CAD build for the part. Positions are in the model's coordinates, mm. A direction names the side the tool comes from. Round coordinates to 2 decimals unless told otherwise and drop trailing zeros. Loops run counter-clockwise (first coordinate to the right, second up) from the corner with the lowest first, then second, coordinate; pieces in that order, holes last.
```python
from build123d import *

# Parameters (mm, degrees)
F0_W      = 73.406
F0_H      = 31.75
F1_DEPTH  = 14.224
F3_DEPTH  = 28.575
F5_DEPTH  = 25.4
F8_DEPTH  = 12.7
F10_DEPTH = 4.826
F12_DEPTH = 4.826


with BuildPart() as f1:
    # F0 (on Front) → F1 (new body, symmetric)
    with BuildSketch(Plane.XZ):
        Rectangle(F0_W, F0_H)
    extrude(amount=F1_DEPTH, both=True)

    # F2 (on face) → F3 (join)
    with BuildSketch(Plane.XY.offset(15.875)):
        Polygon((-36.703, 7.854131), (-36.703, -3.048), (-30.353, -3.048), (-30.353, -7.854131), (32.893, -7.854131), (32.893, -12.7), (67.945, -12.7), (67.945, 12.7), (32.893, 12.7), (32.893, 7.854131), align=None)
    extrude(amount=F3_DEPTH)

    # F4 (on face) → F5 (cut)
    with BuildSketch(Plane.XZ.offset(12.7)):
        Polygon((67.945, 44.45), (37.465, 15.875), (67.945, 15.875), align=None)
    extrude(amount=-F5_DEPTH, mode=Mode.SUBTRACT)

    # F6: F1 across plane


with BuildPart() as f1_1:
    add(f1.part)
    add(f1.part.mirror(Plane.XY))

    # F7 (on Front) → F8 (cut, symmetric)
    with BuildSketch(Plane.XZ):
        with BuildLine():
            ThreePointArc((-6.477, -24.5745), (-10.428313, -26.211187), (-12.065, -30.1625))
            Line((-12.065, -30.1625), (22.987, -30.1625))
            ThreePointArc((22.987, -30.1625), (21.350313, -26.211187), (17.399, -24.5745))
            Line((17.399, -24.5745), (-6.477, -24.5745))
        make_face()
        with BuildLine():
            Line((22.987, -30.1625), (-12.065, -30.1625))
            ThreePointArc((-12.065, -30.1625), (-10.428313, -34.113813), (-6.477, -35.7505))
            Line((-6.477, -35.7505), (17.399, -35.7505))
            ThreePointArc((17.399, -35.7505), (21.350313, -34.113813), (22.987, -30.1625))
        make_face()
        with BuildLine():
            ThreePointArc((-6.477, 35.7505), (-12.065, 30.1625), (-6.477, 24.5745))
            Line((-6.477, 24.5745), (17.399, 24.5745))
            ThreePointArc((17.399, 24.5745), (22.987, 30.1625), (17.399, 35.7505))
            Line((17.399, 35.7505), (-6.477, 35.7505))
        make_face()
    extrude(amount=F8_DEPTH, both=True, mode=Mode.SUBTRACT)

    # F9 (on face) → F10 (cut)
    with BuildSketch(Plane.XZ.offset(12.7)):
        Polygon((32.893, -15.875), (32.893, -26.924), (49.2506, -26.924), (37.465, -15.875), align=None)
        Polygon((37.465, 15.875), (49.2506, 26.924), (32.893, 26.924), (32.893, 15.875), align=None)
    extrude(amount=-F10_DEPTH, mode=Mode.SUBTRACT)

    # F11 (on face) → F12 (cut)
    with BuildSketch(Plane(origin=(0, 12.7, 0), x_dir=(-1, 0, 0), z_dir=(0, 1, 0))):
        Polygon((-49.2506, -26.924), (-32.893, -26.924), (-32.893, -15.875), (-36.703, -15.875), (-37.465, -15.875), align=None)
        Polygon((-37.465, 15.875), (-36.703, 15.875), (-32.893, 15.875), (-32.893, 26.924), (-49.2506, 26.924), align=None)
    extrude(amount=-F12_DEPTH, mode=Mode.SUBTRACT)


solid = f1_1.part
```
Item 1: Cut at B-B, the plane x = -26.5. Give the cut face in (y, z) (3 decimals), plus the area to 3 significant figures.
Answers follow:
outline: (-14.224, -15.875) - (-7.854, -15.875) - (-7.854, -44.45) - (7.854, -44.45) - (7.854, -15.875) - (14.224, -15.875) - (14.224, 15.875) - (7.854, 15.875) - (7.854, 44.45) - (-7.854, 44.45) - (-7.854, 15.875) - (-14.224, 15.875) - close
area: 1,800 mm2
Item 2: Cut at C-C, the plane x = 55. Give the cut face in (y, z), plus the area to 3 significant figures.
Answers follow:
outline: (-12.7, -44.45) - (12.7, -44.45) - (12.7, -32.31) - (-12.7, -32.31) - close; (-12.7, 32.31) - (12.7, 32.31) - (12.7, 44.45) - (-12.7, 44.45) - close
area: 617 mm2
Item 3: Two-plate mould, pull along X, no slides. Class faces 4 (the flat face through (32.893, 10, 36)), 5 (the flat face through (27, 0, -44.45)), 6 (the flat face through (5, 0, -35.75)): released by +X, released by -X, zero draft, split by the parting line, or undercut.
Answers follow:
face 4: released by -X
face 5: zero draft
face 6: undercut
Item 4: Cut at A-A, the plane y = 11. Give the cut face in (x, z) (3 decimals), plus the area to 3 significant figures.
Answers follow:
outline: (-36.703, -15.875) - (36.703, -15.875) - (36.703, 15.875) - (-36.703, 15.875) - close; (32.893, -44.45) - (67.945, -44.45) - (49.251, -26.924) - (32.893, -26.924) - close; (32.893, 26.924) - (49.251, 26.924) - (67.945, 44.45) - (32.893, 44.45) - close
area: 3,230 mm2
Item 5: Probe line 1 (Z direction, x = -1, y = -4.5); line 2 (X direction, y = 6.75, z = -7); line 3 (Y direction, x = -14, z = -39). List the from-to ranges inside material, lowest first.
Answers follow:
line 1: z = -44.45 to -35.75, -24.57 to 24.57, 35.75 to 44.45
line 2: x = -36.7 to 36.7
line 3: y = -7.85 to 7.85
Item 6: Cut at D-D, the plane y = 0.75. State how many separate pieces and enclosed holes the cut face has, plus the area to 3 significant figures.
Answers follow:
separate pieces: 1
enclosed holes: 2
area: 6,710 mm2
Item 7: Flat gauge pins, fed straight in: P1, Ø4, axis at y = -11, z = 24.5, coming from the -X side; P2, Ø3, axis at x = 3, y = 10.5, coming from the +Z side (3 decimals); P3, Ø4, axis at y = -5.5, z = -31.5, coming from the -X side; P4, Ø19.5, axis at x = 55, z = -39, coming from the -Y side. Where does each tip first touch, or does it go through?
Answers follow:
P1: passes through
P2: stops at z = 15.875
P3: stops at x = -30.35
P4: stops at y = -12.7
Item 8: 3-axis set-ups, long thin cutter, end or side, ignore diameter. For faces 1 (the flat face through (5, 0, 24.574)), 2 (the flat face through (39, -7.874, 23)), 3 (the flat face through (-34, -3.048, -30)): which of +Z, -Z, +X, -X, +Y, -Y reach the whole face in a straight line?
Answers follow:
face 1: +Y, -Y
face 2: +X, -X, -Y
face 3: -Z, -X, -Y
